from build123d import *

# Parameters (mm, degrees)
F0_R     = 25.81628
F1_DEPTH = 3
F3_DEPTH = 25
F5_DEPTH = 25


with BuildPart() as f1:
    # F0 (on Front) → F1 (new body)
    with BuildSketch(Plane.XZ):
        Circle(F0_R)
    extrude(amount=F1_DEPTH)

    # F2 (on face) → F3 (cut)
    with BuildSketch(Plane.XZ.offset(3)):
        Polygon((-22.232322, 11.412702), (-22.232322, -11.196028), (-20.024735, -14.393222), (-20.024735, 13.163546), align=None)
        Polygon((-11.118267, 22.146139), (-13.630347, 19.329563), (-14.010966, -19.569632), (-11.118267, -22.157835), align=None)
        Polygon((-6.170227, 24.353726), (-9.215174, 22.755129), (-9.671916, -22.61458), (-6.170227, -23.832556), align=None)
        Polygon((-0.765447, -24.51767), (-0.765447, 25.038838), (-5.028372, 24.277601), (-5.028372, -24.51767), align=None)
        Polygon((5.443127, -23.527138), (6.052805, 24.129314), (1.276998, 25.038838), (1.276998, -24.51767), align=None)
        Polygon((12.251193, 21.588992), (7.98345, 23.113187), (7.092044, -22.985913), (10.320548, -22.409394), align=None)
        Polygon((17.026998, 17.62609), (13.876999, 20.064799), (13.876999, 19.251894), (11.844741, -21.49488), (14.893129, -19.869074), align=None)
        Polygon((20.731321, 13.848901), (18.551191, 15.695445), (16.85815, -18.250049), (19.262481, -15.60133), align=None)
        Polygon((23.631837, 8.277702), (22.209259, 6.143831), (20.9899, -12.04488), (22.920547, -9.504557), align=None)
    extrude(amount=-F3_DEPTH, mode=Mode.SUBTRACT)

    # F4 (on face) → F5 (cut)
    with BuildSketch(Plane.XZ.offset(3)):
        Polygon((-15.8276, 18.478015), (-18.247107, 15.816556), (-18.547006, -14.833115), (-15.8276, -17.733933), align=None)
    extrude(amount=-F5_DEPTH, mode=Mode.SUBTRACT)


solid = f1.part
Can you work these out from the model? Positions are in its coordinate system, mm. Round coordinates to 2 decimals unless told otherwise and drop trailing zeros. Order: outer loops, then holes, each group sorted by start corner. A loop starts at its lowest first (then second) coordinate and runs counter-clockwise, first axis right, second up. Notation, with made-up numbers: (85.5, -38.5) -> (131.5, -38.5) arc R14 cw to (131.5, -14.5) -> close; hole circle Ø6 at (8.25, 47). An arc over 180 degrees is marked (long way). Write each question's results on one line, items separated by ' | '. Start each with the question number.
Item 1: If we section it at A-A, the plane x = -12.5: Write out the boundary of the cut face in (y, z).
Item 2: If we section it at B-B, the plane z = 5: State how many separate pieces and enclosed holes the cut face has, then the cut area to 3 significant figures.
Item 3: Will these pins go through, and if not, where does the flat tip stop? pin 1 (0.9 mm diameter, centred on y = -1.5, z = 10, fed in from -X); pin 2 (1 mm diameter, centred on x = -17, y = -1.5, fed in from -Z); pin 3 (1.5 mm diameter, centred on x = -3, y = -1.5, fed in from +Z).
Item 4: Please list where these lines run through material, in increasing order: L1, parallel to Z at x = -20.5, y = -0.6; L2, parallel to Z at x = 1, y = -1.35; L3, parallel to Z at x = -17, y = -1.05.
Item 5: If we section it at C-C, the plane x = -3: Write out the boundary of the cut face in (y, z).
Results:
1) outline: (-3, -22.59) -> (0, -22.59) -> (0, -20.92) -> (-3, -20.92) -> close; (-3, 20.6) -> (0, 20.6) -> (0, 22.59) -> (-3, 22.59) -> close
2) separate pieces: 11 | enclosed holes: 0 | area: 61.7 mm2
3) pin 1: stops at x = -23.98 | pin 2: stops at z = -19.86 | pin 3: stops at z = 25.72
4) L1: z = -15.69 to -13.7, 12.79 to 15.69 | L2: z = -25.8 to 25.8 | L3: z = -19.43 to -16.48, 17.19 to 19.43
5) outline: (-3, -25.64) -> (0, -25.64) -> (0, -24.52) -> (-3, -24.52) -> close; (-3, 24.64) -> (0, 24.64) -> (0, 25.64) -> (-3, 25.64) -> close
